Geometry check sheet. Reference: the model listing, model coordinates, mm. Face numbers are marked on the shaded views. A direction names the side the tool comes from. Round coordinates to 2 decimals unless told otherwise and drop trailing zeros. Write each loop counter-clockwise with the first axis right and the second up, starting at its lowest first coordinate (ties: lowest second). Pieces come first, ordered by that corner, then holes.
Item 1: Cross-section at D-D (x = -1104.75). Enter the section's corners in (y, z).
Item 2: Cross-section at C-C (x = -1099). Enter the section's corners in (y, z).
Item 3: Draft check along X on the marked faces 3, 4, 5 and 6. Enter one of: pulls with the +X half, pulls with the -X half, needs draft (parallel to the pull), parting line crosses it, or undercut.
Item 4: Depth check by flat-ended pin: P1, Ø9, axis at x = -1098.5, y = 80.5, coming from the +Z side; P2, Ø2, axis at x = -1106.5, y = 81.5, coming from the +Z side; P3, Ø12, axis at x = -1105, z = 76.5, coming from the +Y side. Enter the tip coordinate at first touch or a pass-through.
Item 5: Access from +Z, -Z, +X, -X, +Y, -Y to the whole of each face (thin tool, end or side, straight path). Record for the marked faces 1 and 2.
Item 6: Cross-section at A-A (z = 40). Enter the section's corners in (x, y).
Item 7: Cross-section at B-B (x = -1090). Enter the section's corners in (y, z).
Item 8: Scan lines: probe 1 along X at (y, z) = (88.25, 39); probe 2 along Z at (x, y) = (-1101.75, 84); probe 3 along X at (y, z) = (76.75, 68). Record each from-to range of solid material in increasing order.
from build123d import *

# Parameters (mm, degrees)
SKETCH1_R           = 1.6
BOSS_EXTRUDE1_DEPTH = 2.5
SKETCH2_R           = 1.6
BOSS_EXTRUDE2_DEPTH = 4
SKETCH3_W           = 23
SKETCH3_H           = 20
BOSS_EXTRUDE3_DEPTH = 8
FILLET1_R           = 3
FILLET2_R           = 15
FILLET3_R           = 2


with BuildPart() as part:
    # Sketch1 → Boss-Extrude1 (new, symmetric)
    with BuildSketch(Plane.ZY.offset(1089.950719415)):
        with BuildLine():
            Line((82.004058992, 86.47718844), (82.004058992, 83.796629248))
            ThreePointArc((82.004058992, 83.796629248), (80.970825694, 80.752822103), (78.298154218, 78.967000116))
            Line((78.298154218, 78.967000116), (64.004058992, 75.136908844))
            Line((64.004058992, 75.136908844), (27.004058992, 75.136908844))
            Line((27.004058992, 75.136908844), (27.004058992, 95.136908844))
            Line((27.004058992, 95.136908844), (64.004058992, 95.136908844))
            Line((64.004058992, 95.136908844), (78.298154218, 91.306817572))
            ThreePointArc((78.298154218, 91.306817572), (80.970825694, 89.520995585), (82.004058992, 86.47718844))
        make_face()
        with Locations((72.667931354, 85.136908844)):
            Circle(SKETCH1_R, mode=Mode.SUBTRACT)
    extrude(amount=BOSS_EXTRUDE1_DEPTH, both=True)



with BuildPart() as body_2:
    # Sketch2 → Boss-Extrude2 (new body)
    with BuildSketch(Plane.ZY.offset(1106.450719415)):
        with BuildLine():
            Line((27.004058992, 95.136908844), (27.004058992, 75.136908844))
            Line((27.004058992, 75.136908844), (64.004058992, 75.136908844))
            Line((64.004058992, 75.136908844), (78.298154218, 78.967000116))
            ThreePointArc((78.298154218, 78.967000116), (80.970825694, 80.752822103), (82.004058992, 83.796629248))
            Line((82.004058992, 83.796629248), (82.004058992, 86.47718844))
            ThreePointArc((82.004058992, 86.47718844), (80.970825694, 89.520995585), (78.298154218, 91.306817572))
            Line((78.298154218, 91.306817572), (64.004058992, 95.136908844))
            Line((64.004058992, 95.136908844), (27.004058992, 95.136908844))
        make_face()
        with Locations((72.667931354, 85.136908844)):
            Circle(SKETCH2_R, mode=Mode.SUBTRACT)
    extrude(amount=BOSS_EXTRUDE2_DEPTH)


with BuildPart() as part_1:
    add(part.part)

    add(body_2.part)  # Boss-Extrude3 merges body 2
    # Sketch3 → Boss-Extrude3 (add)
    with BuildSketch(Plane(origin=(0, 0, 27.004058992), x_dir=(-1, 0, 0), z_dir=(0, 0, -1))):
        with Locations((1098.950719415, 85.136908844)):
            Rectangle(SKETCH3_W, SKETCH3_H)
    extrude(amount=-BOSS_EXTRUDE3_DEPTH)

    # Fillet1
    fillet1_edges = [part_1.edges().sort_by_distance(p)[0] for p in [
        (-1092.450719415, 85.136908844, 35.004058992),
        (-1106.450719415, 85.136908844, 35.004058992),
    ]]
    fillet(fillet1_edges, radius=FILLET1_R)

    # Fillet2
    fillet2_edges = [part_1.edges().sort_by_distance(p)[0] for p in [
        (-1089.950719415, 95.136908844, 64.004058992),
        (-1089.950719415, 75.136908844, 64.004058992),
        (-1108.450719415, 95.136908844, 64.004058992),
        (-1108.450719415, 75.136908844, 64.004058992),
    ]]
    fillet(fillet2_edges, radius=FILLET2_R)

    # Fillet3
    fillet3_edges = [part_1.edges().sort_by_distance(p)[0] for p in [
        (-1087.450719415, 80.752822103, 80.970825694),
        (-1087.450719415, 75.136908844, 44.51666526),
        (-1110.450719415, 80.752822103, 80.970825694),
        (-1110.450719415, 85.136908844, 82.004058992),
        (-1110.450719415, 89.520995585, 80.970825694),
        (-1110.450719415, 92.966306905, 72.104855711),
        (-1110.450719415, 95.136908844, 44.51666526),
        (-1087.450719415, 95.136908844, 44.51666526),
        (-1087.450719415, 92.966306905, 72.104855711),
        (-1110.450719415, 75.136908844, 44.51666526),
        (-1087.450719415, 89.520995585, 80.970825694),
        (-1110.450719415, 77.307510783, 72.104855711),
        (-1110.450719415, 75.265235923, 63.987164412),
        (-1110.450719415, 95.008581765, 63.987164412),
        (-1087.450719415, 77.307510783, 72.104855711),
        (-1087.450719415, 75.265235923, 63.987164412),
        (-1087.450719415, 95.008581765, 63.987164412),
        (-1087.450719415, 85.136908844, 82.004058992),
    ]]
    fillet(fillet3_edges, radius=FILLET3_R)


solid = part_1.part
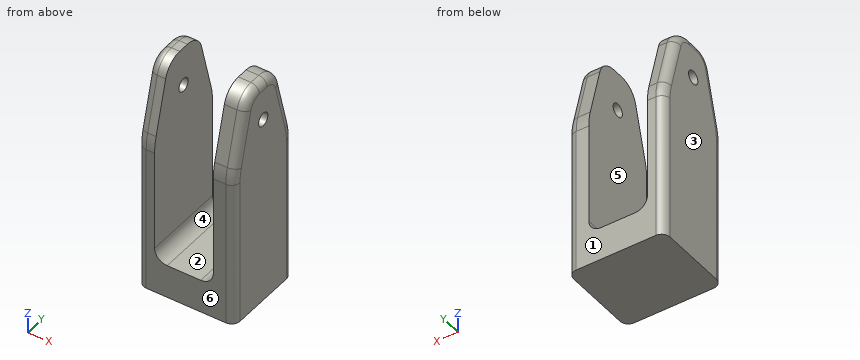
Resolved:
1. outline: (75.14, 27) - (95.14, 27) - (95.14, 35.3) - (75.14, 35.3) - close
2. outline: (75.14, 27) - (95.14, 27) - (95.14, 35) - (75.14, 35) - close
3. face 3: pulls with the -X half
3. face 4: undercut
3. face 5: undercut
3. face 6: needs draft
4. P1: stops at z = 35.38
4. P2: stops at z = 81.83
4. P3: stops at y = 93.35
5. face 1: +Z, -Z, +X, -X, +Y
5. face 2: +Z, +Y, -Y
6. outline: (-1110.45, 77.14) arc R2 ccw to (-1108.45, 75.14) - (-1106.45, 75.14) - (-1106.45, 95.14) - (-1108.45, 95.14) arc R2 ccw to (-1110.45, 93.14) - close; (-1092.45, 75.14) - (-1089.45, 75.14) arc R2 ccw to (-1087.45, 77.14) - (-1087.45, 93.14) arc R2 ccw to (-1089.45, 95.14) - (-1092.45, 95.14) - close
7. outline: (75.14, 27) - (95.14, 27) - (95.14, 62.03) arc R15 ccw to (94.63, 65.91) - (91.31, 78.3) arc R5 ccw to (86.48, 82) - (83.8, 82) arc R5 ccw to (78.97, 78.3) - (75.65, 65.91) arc R15 ccw to (75.14, 62.03) - close; hole circle Ø3.2 at (85.14, 72.67)
8. probe 1: x = -1110.45 to -1106.45, -1092.45 to -1087.45
8. probe 2: z = 27 to 35
8. probe 3: x = -1109.8 to -1106.45, -1092.45 to -1088.1
